from build123d import *

# Parameters (mm, degrees)
SKETCH2_W           = 27.3
SKETCH2_H           = 30
BOSS_EXTRUDE1_DEPTH = 6.35
SKETCH3_W           = 12.7
SKETCH3_H           = 6.35
BOSS_EXTRUDE2_DEPTH = 6.35
SKETCH4_R           = 3.075
CUT_EXTRUDE1_DEPTH  = 7.35
CUT_EXTRUDE2_REACH  = 32
SKETCH5_W           = 3.2
SKETCH5_H           = 6.35


with BuildPart() as part:
    # Sketch2 → Boss-Extrude1 (new body)
    with BuildSketch(Plane(origin=(0, 0, 0), x_dir=(1, 0, 0), z_dir=(0, 1, 0))):
        Rectangle(SKETCH2_W, SKETCH2_H)
    extrude(amount=BOSS_EXTRUDE1_DEPTH)

    # Sketch3 → Boss-Extrude2 (add)
    with BuildSketch(Plane(origin=(13.65, 0, 0), x_dir=(0, 0, -1), z_dir=(1, 0, 0))):
        with Locations((0, 3.175)):
            Rectangle(SKETCH3_W, SKETCH3_H)
    boss_extrude2 = extrude(amount=BOSS_EXTRUDE2_DEPTH)

    # Mirror1: Boss-Extrude2 across plane
    add(boss_extrude2.mirror(Plane(origin=(0, 0, 0), x_dir=(0, 0, 1), z_dir=(1, 0, 0))))

    # Sketch4 → Cut-Extrude1 (cut, through all)
    with BuildSketch(Plane(origin=(0, 6.35, 0), x_dir=(1, 0, 0), z_dir=(0, 1, 0))):
        Circle(SKETCH4_R)
    extrude(amount=-CUT_EXTRUDE1_DEPTH, mode=Mode.SUBTRACT)

    # Sketch5 → Cut-Extrude2 (cut, up to next)
    with BuildSketch(Plane.XY.offset(15), mode=Mode.PRIVATE) as cut_extrude2_sk1:
        with Locations((0, 3.175)):
            Rectangle(SKETCH5_W, SKETCH5_H)
    cut_extrude2_tool1 = extrude(cut_extrude2_sk1.sketch, amount=-CUT_EXTRUDE2_REACH, mode=Mode.PRIVATE) & part.part
    add(cut_extrude2_tool1.solids().sort_by_distance((0, 3.175, 15))[0], mode=Mode.SUBTRACT)


solid = part.part
Input: part model. Units: mm. Frame: model coordinates. A direction names the side the tool comes from. Coordinates: 2 decimals unless noted, no trailing zeros. Loops run counter-clockwise (first coordinate to the right, second up) from the corner with the lowest first, then second, coordinate; pieces in that order, holes last. Notation, with made-up numbers: (36, 80) -> (69, 80) arc R26 cw to (69, 102) -> close; hole circle Ø5 at (22.5, 87.25). An arc over 180 degrees is marked (long way). Write item = value, one per line. Start each with the question number.
Item 1: Material intervals for line 1 (X direction, y = 1.5, z = 0) (3 decimals); line 2 (Z direction, x = 0, y = 2.25) (3 decimals); line 3 (X direction, y = 5.25, z = 1.75), sorted ascending.
Item 2: Mould query, pull axis Z, two halves, no side actions, for faces 1 (the face through (-8, 3, 15)), 2 (the face through (17, 3, -6.35)), 3 (the face through (0.112, 3.219, -3.073)), 4 (the face through (-13.65, 3, -11)). Classes: pulls with the +Z half, pulls with the -Z half, needs draft (parallel to the pull), parting line crosses it, or undercut.
Item 3: Cut plane B-B, the plane y = 3.75. Return loops of the section in (x, z) (3 decimals).
Item 4: Cut plane C-C, the plane z = 0. Return loops of the section in (x, y) (3 decimals), plus the area to 3 significant figures.
Item 5: Reachability of faces 5 (the face through (17, 3, 6.35)), 6 (the face through (-1.6, 3, 9)), 7 (the face through (13.65, 3, -11)) from +Z, -Z, +X, -X, +Y, -Y: full face, straight path, thin tool, end or side. Return the list, or none.
Item 6: Cut plane D-D, the plane x = 0. Return loops of the section in (y, z) (3 decimals), plus the area to 3 significant figures.
Item 7: Cut plane A-A, the plane z = 13.25. Return loops of the section in (x, y).
Item 8: First-contact query: P1, Ø2, axis at y = 3, z = -7.5, coming from the -X side; P2, Ø1.9, axis at y = 2.5, z = 9, coming from the +X side; P3, Ø1.9, axis at x = -18, y = 4, coming from the -Z side. Flat tips, straight axial feed; report the tip coordinate or a pass-through.
Ans:
q1.line_1 = -20 to -3.075, 3.075 to 20
q1.line_2 = -15 to -3.075
q1.line_3 = -20 to -2.53, 2.53 to 20
q2.face_1 = pulls with the +Z half
q2.face_2 = pulls with the -Z half
q2.face_3 = undercut
q2.face_4 = needs draft
q3.outline = (-20, -6.35) -> (-13.65, -6.35) -> (-13.65, -15) -> (13.65, -15) -> (13.65, -6.35) -> (20, -6.35) -> (20, 6.35) -> (13.65, 6.35) -> (13.65, 15) -> (1.6, 15) -> (1.6, 2.626) arc R3.075 cw (long way) to (-1.6, 2.626) -> (-1.6, 15) -> (-13.65, 15) -> (-13.65, 6.35) -> (-20, 6.35) -> close
q4.outline = (-20, 0) -> (-3.075, 0) -> (-3.075, 6.35) -> (-20, 6.35) -> close; (3.075, 0) -> (20, 0) -> (20, 6.35) -> (3.075, 6.35) -> close
q4.area = 215 mm²
q5.face_5 = +Z, +X, +Y, -Y
q5.face_6 = +Z, +Y, -Y
q5.face_7 = -Z, +X, +Y, -Y
q6.outline = (0, -15) -> (6.35, -15) -> (6.35, -3.075) -> (0, -3.075) -> close
q6.area = 75.7 mm²
q7.outline = (-13.65, 0) -> (-1.6, 0) -> (-1.6, 6.35) -> (-13.65, 6.35) -> close; (1.6, 0) -> (13.65, 0) -> (13.65, 6.35) -> (1.6, 6.35) -> close
q8.P1 = -13.65
q8.P2 = 13.65
q8.P3 = -6.35
